Solid Edge part; units mm, degrees
sketch "Sketch1" plane through (0, 0, 0) normal (0, -1, 0) x (1, 0, 0)
  line L0 (-1.3, 0) -> (-1.3, -1.3365)
  arc A0 (-1.3, -1.3365) -> (-0.7523, -1.9342) centre (-0.7, -1.3365) ccw
  line L1 (-0.7523, -1.9342) -> (0, -2)
  line L2 (0, -2) -> (0, -0.8545)
  arc A1 (0, -0.8545) -> (0.1, -0.7545) centre (0.1, -0.8545) cw
  line L3 (0.1, -0.7545) -> (0.5545, -0.7545)
  line L4 (0.5545, -0.7545) -> (0.8, -1)
  line L5 (0.8, -1) -> (5.6931, -1)
  line L6 (5.6931, -1) -> (6, -0.6931)
  line L7 (6, -0.6931) -> (6, 0)
  line L8 (6, 0) -> (-1.3, 0)
revolve "RevolvedProtrusion1" add sketch "Sketch1" angle 360 about axis through (6, 0, 0) along (-1, 0, 0)
sketch "Sketch2" plane through (0, 0, 0) normal (0, 0, 1) x (1, 0, 0)
  line L0 (-2.3, 0.25) -> (-2.3, -0.25)
  line L1 (-2.3, -0.25) -> (-0.8, -0.25)
  line L2 (-0.8, -0.25) -> (-0.8, 0.25)
  line L3 (-0.8, 0.25) -> (-2.3, 0.25)
extrude "ExtrudedCutout_1" cut sketch "Sketch2" against normal blind 2.6 and the other way blind 2.6
properties part number "bene_inox_210211-2X6"
Verification items for the finished model (mm, model axes). Round coordinates to 2 decimals unless told otherwise and drop trailing zeros. Write each loop counter-clockwise with the first axis right and the second up, starting at its lowest first coordinate (ties: lowest second). Pieces come first, ordered by that corner, then holes.
1. Section check D-D on x = 2.5. Enter the section's corners in (y, z).
2. Draft check along X on faces 1 (the flat face through (-1.3, -1, 0)), 2 (the cylindrical face through (3, -1, 0)), 3 (the flat face through (6, 0, 0)), 4 (the cylindrical face through (0.33, -0.737, 0.164)). Enter one of: +X half, -X half, draft (parallel to the pull), parting line (faces both ways), or undercut.
3. Gauge pin test, flat end, axial feed: P1, Ø1.5, axis at x = 2.5, z = -1, coming from the -Y side. Record the tip position at first contact, or that the pin passes through.
4. Section check C-C on x = 0.25. Enter the section's corners in (y, z), plus the area to 3 significant figures.
5. Scan lines: L1, parallel to X at y = -0.85, z = -1.05; L2, parallel to X at y = -0.4, z = -0.7; L3, parallel to Z at x = 3.75, y = -0.6. Record each from-to range of solid material in increasing order.
6. Section check B-B on y = 0. Enter the section's corners in (x, z).
7. Section check A-A on z = 0. Enter the section's corners in (x, y), plus the area to 3 significant figures.
Answer:
1. outline: circle Ø2 at (0, 0)
2. face 1: -X half
2. face 2: draft
2. face 3: +X half
2. face 4: undercut
3. P1: stops at y = -0.97
4. outline: circle Ø1.51 at (0, 0)
4. area: 1.79 mm2
5. L1: x = -1.3 to 0
5. L2: x = -1.3 to 0.01, 0.61 to 5.89
5. L3: z = -0.8 to 0.8
6. outline: (-0.8, -1.93) arc R0.6 ccw to (-0.75, -1.93) - (0, -2) - (0, -0.85) arc R0.1 cw to (0.1, -0.75) - (0.55, -0.75) - (0.8, -1) - (5.69, -1) - (6, -0.69) - (6, 0.69) - (5.69, 1) - (0.8, 1) - (0.55, 0.75) - (0.1, 0.75) arc R0.1 cw to (0, 0.85) - (0, 2) - (-0.75, 1.93) arc R0.6 ccw to (-0.8, 1.93) - close
7. outline: (-1.3, -1.34) arc R0.6 ccw to (-0.75, -1.93) - (0, -2) - (0, -0.85) arc R0.1 cw to (0.1, -0.75) - (0.55, -0.75) - (0.8, -1) - (5.69, -1) - (6, -0.69) - (6, 0.69) - (5.69, 1) - (0.8, 1) - (0.55, 0.75) - (0.1, 0.75) arc R0.1 cw to (0, 0.85) - (0, 2) - (-0.75, 1.93) arc R0.6 ccw to (-1.3, 1.34) - (-1.3, 0.25) - (-0.8, 0.25) - (-0.8, -0.25) - (-1.3, -0.25) - close
7. area: 16.3 mm2
